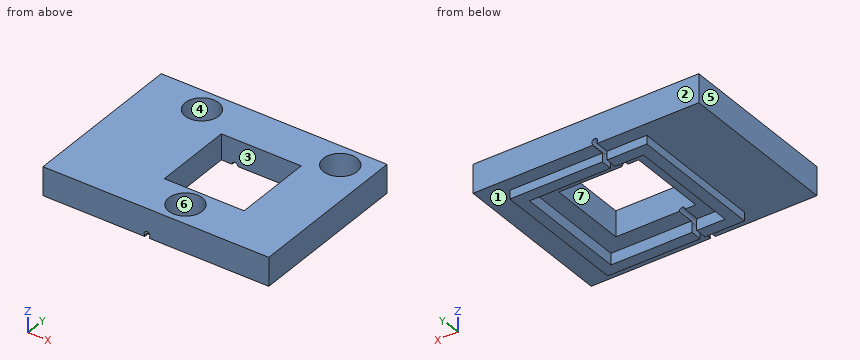
Autodesk Inventor part; units mm, degrees
ref_plane "YZ Plane" through (0, 0, 0) normal (1, 0, 0) x (0, 1, 0)
ref_plane "XZ Plane" through (0, 0, 0) normal (0, 1, 0) x (-1, 0, 0)
ref_plane "XY Plane" through (0, 0, 0) normal (0, 0, 1) x (1, 0, 0)
ref_plane "Work Plane1" through (52.5141, 202.7033, 6.4479) normal (0, 0, -1) x (0, 1, 0)
sketch "Sketch1" plane through (52.5141, 202.7033, 6.4479) normal (0, 0, -1) x (0, 1, 0)
  circle A0 centre (-59.8114, -30.5) radius 1.4 construction
  circle A1 centre (-38.8114, -18.3756) radius 1.4
  circle A2 centre (-38.8114, -42.6244) radius 1.4 construction
  circle A3 centre (41, 0) radius 1.65
  circle A4 centre (-9, 0) radius 1.65
  circle A5 centre (-9, 50) radius 1.65
  circle A6 centre (41, 50) radius 1.65
  circle A7 centre (16, 50) radius 1.65
  circle A8 centre (-9, 25) radius 1.65
  circle A9 centre (16, 0) radius 1.65
  circle A10 centre (41, 25) radius 1.65
  line L0 (80, 55) -> (-80, 55)
  line L1 (-80, 55) -> (-80, -55)
  line L2 (-80, -55) -> (80, -55)
  line L3 (80, -55) -> (80, 55)
  line L4 (-36.5, 0) -> (-36.5, -50)
  line L5 (-14, 0) -> (-36.5, 0)
  line L6 (-14, -5) -> (-14, 0)
  line L7 (72, -5) -> (-14, -5)
  line L8 (72, -50) -> (72, -5)
  line L9 (-36.5, -50) -> (72, -50)
  line L10 (-4, 45) -> (-4, 5)
  line L11 (36, 45) -> (-4, 45)
  line L12 (36, 5) -> (36, 45)
  line L13 (-4, 5) -> (36, 5)
  line L14 (-64.5989, -17.0433) -> (-64.5989, -57.0433) construction
  line L15 (-64.5989, -57.0433) -> (-34.5989, -57.0433) construction
  line L16 (-34.5989, -57.0433) -> (-34.5989, -17.0433) construction
  line L17 (-34.5989, -17.0433) -> (-64.5989, -17.0433) construction
  line L18 (-34.8114, -13.0433) -> (-63.8114, -13.0433)
  line L19 (-63.8114, -13.0433) -> (-63.8114, -52.6244)
  line L20 (-63.8114, -52.6244) -> (-34.8114, -52.6244)
  line L21 (-34.8114, -52.6244) -> (-34.8114, -13.0433)
  circle A11 centre (-59.8114, -30.5) radius 2.95
  circle A12 centre (-38.8114, -18.3756) radius 2.95
  circle A13 centre (-38.8114, -42.6244) radius 2.95 construction
  line L22 (-36.5, -35.1157) -> (-41.75, -35.1157) construction
  line L23 (-41.75, -35.1157) -> (-41.75, -38.5657) construction
  line L24 (-41.75, -38.5657) -> (-56.86, -38.5657) construction
  line L25 (-56.86, -38.5657) -> (-56.86, -35.1157) construction
  line L26 (-56.86, -35.1157) -> (-60.26, -35.1157) construction
  line L27 (-60.26, -35.1157) -> (-60.26, -52.0657) construction
  line L28 (-60.26, -52.0657) -> (-36.5, -52.0657) construction
  line L29 (-36.5, -52.0657) -> (-36.5, -35.1157) construction
  line L30 (-41.75, -28.3657) -> (-36.5, -28.3657) construction
  line L31 (-36.5, -28.3657) -> (-36.5, -25.0657) construction
  line L32 (-36.5, -25.0657) -> (-60.26, -25.0657) construction
  line L33 (-60.26, -25.0657) -> (-60.26, -28.3657) construction
  line L34 (-60.26, -28.3657) -> (-56.86, -28.3657) construction
  line L35 (-56.86, -28.3657) -> (-56.86, -27.0942) construction
  line L36 (-56.86, -27.0942) -> (-41.75, -27.0942) construction
  line L37 (-41.75, -27.0942) -> (-41.75, -28.3657) construction
  line L38 (-56.86, -35.1157) -> (-60.26, -35.1157) construction
  line L39 (-56.86, -38.5657) -> (-56.86, -35.1157) construction
  line L40 (-41.75, -38.5657) -> (-56.86, -38.5657) construction
  line L41 (-41.75, -35.1157) -> (-41.75, -38.5657) construction
  line L42 (-36.5, -35.1157) -> (-41.75, -35.1157) construction
  line L43 (-36.5, -35.05) -> (-36.5, -35.1157) construction
  line L44 (-36.5, -35.05) -> (-56.86, -35.05) construction
  line L45 (-36.5, -34.78) -> (-36.5, -35.05) construction
  line L46 (-36.5, -34.78) -> (-56.86, -34.78) construction
  line L47 (-36.5, -34.51) -> (-36.5, -34.78) construction
  line L48 (-36.5, -34.51) -> (-56.86, -34.51) construction
  line L49 (-36.5, -34.24) -> (-36.5, -34.51) construction
  line L50 (-36.5, -34.24) -> (-56.86, -34.24) construction
  line L51 (-36.5, -33.97) -> (-36.5, -34.24) construction
  line L52 (-36.5, -33.97) -> (-56.86, -33.97) construction
  line L53 (-36.5, -33.7) -> (-36.5, -33.97) construction
  line L54 (-36.5, -33.7) -> (-56.86, -33.7) construction
  line L55 (-36.5, -33.43) -> (-36.5, -33.7) construction
  line L56 (-36.5, -33.43) -> (-56.86, -33.43) construction
  line L57 (-36.5, -33.16) -> (-36.5, -33.43) construction
  line L58 (-36.5, -33.16) -> (-56.86, -33.16) construction
  line L59 (-36.5, -32.89) -> (-36.5, -33.16) construction
  line L60 (-36.5, -32.89) -> (-56.86, -32.89) construction
  line L61 (-36.5, -32.62) -> (-36.5, -32.89) construction
  line L62 (-36.5, -32.62) -> (-56.86, -32.62) construction
  line L63 (-36.5, -32.35) -> (-36.5, -32.62) construction
  line L64 (-36.5, -32.35) -> (-56.86, -32.35) construction
  line L65 (-36.5, -32.08) -> (-36.5, -32.35) construction
  line L66 (-36.5, -32.08) -> (-56.86, -32.08) construction
  line L67 (-36.5, -31.81) -> (-36.5, -32.08) construction
  line L68 (-36.5, -31.81) -> (-56.86, -31.81) construction
  line L69 (-36.5, -31.54) -> (-36.5, -31.81) construction
  line L70 (-36.5, -31.54) -> (-56.86, -31.54) construction
  line L71 (-36.5, -31.27) -> (-36.5, -31.54) construction
  line L72 (-36.5, -31.27) -> (-56.86, -31.27) construction
  line L73 (-36.5, -31) -> (-36.5, -31.27) construction
  line L74 (-36.5, -31) -> (-56.86, -31) construction
  line L75 (-36.5, -30.73) -> (-36.5, -31) construction
  line L76 (-36.5, -30.73) -> (-56.86, -30.73) construction
  line L77 (-36.5, -30.46) -> (-36.5, -30.73) construction
  line L78 (-36.5, -30.46) -> (-56.86, -30.46) construction
  line L79 (-36.5, -30.19) -> (-36.5, -30.46) construction
  line L80 (-36.5, -30.19) -> (-56.86, -30.19) construction
  line L81 (-36.5, -29.92) -> (-36.5, -30.19) construction
  line L82 (-36.5, -29.92) -> (-56.86, -29.92) construction
  line L83 (-36.5, -29.65) -> (-36.5, -29.92) construction
  line L84 (-36.5, -29.65) -> (-56.86, -29.65) construction
  line L85 (-36.5, -29.38) -> (-36.5, -29.65) construction
  line L86 (-36.5, -29.38) -> (-56.86, -29.38) construction
  line L87 (-36.5, -29.11) -> (-36.5, -29.38) construction
  line L88 (-36.5, -29.11) -> (-56.86, -29.11) construction
  line L89 (-36.5, -28.84) -> (-36.5, -29.11) construction
  line L90 (-36.5, -28.84) -> (-56.86, -28.84) construction
  line L91 (-36.5, -28.3657) -> (-36.5, -28.84) construction
  line L92 (-41.75, -28.3657) -> (-36.5, -28.3657) construction
  line L93 (-41.75, -27.0942) -> (-41.75, -28.3657) construction
  line L94 (-56.86, -27.0942) -> (-41.75, -27.0942) construction
  line L95 (-56.86, -28.3657) -> (-56.86, -27.0942) construction
  line L96 (-60.26, -28.3657) -> (-56.86, -28.3657) construction
  line L97 (-60.26, -35.1157) -> (-60.26, -28.3657) construction
  line L98 (-60.26, -25.0657) -> (-36.5, -25.0657) construction
  line L99 (-36.5, -25.0657) -> (-36.5, -52.0657) construction
  line L100 (-60.26, -52.0657) -> (-60.26, -25.0657) construction
  line L101 (-57.1632, -22.5233) -> (-33.4032, -22.5233) construction
  line L102 (-33.4032, -22.5233) -> (-33.4032, -49.5233) construction
  line L103 (-33.4032, -49.5233) -> (-57.1632, -49.5233) construction
  line L104 (-57.1632, -49.5233) -> (-57.1632, -22.5233) construction
  circle A14 centre (-38.8114, -42.6244) radius 2.95
  point P0 (-202.7033, -52.5141)
  point P1 (-56.7146, -27.9576)
  dimension "d0" = 4
  dimension "d2" = 4
  dimension "d3" = 4
  dimension "d4" = 5.9
  dimension "d5" = 5.9
  dimension "d6" = 5.9
  dimension "d10" = 10
extrude "Extrusion1" add sketch "Sketch1" along normal blind 2.5 contours L18 L21 L9 L4 A14 A12 | L4 A12 A14 L9 L21 L20 L19 L18
sketch "Sketch2" plane through (52.5141, 202.7033, 3.9479) normal (0, 0, -1) x (-1, 0, 0)
  circle A0 centre (42.6244, -38.8114) radius 2.95
  circle A1 centre (18.3756, -38.8114) radius 2.95
  circle A2 centre (30.5, -59.8114) radius 2.95
  line L0 (13.0433, -34.8114) -> (13.0433, -63.8114)
  line L1 (13.0433, -63.8114) -> (52.6244, -63.8114)
  line L2 (52.6244, -63.8114) -> (52.6244, -34.8114)
  line L3 (52.6244, -34.8114) -> (13.0433, -34.8114)
  point P0 (52.5141, -202.7033)
extrude "Extrusion2" add sketch "Sketch2" along normal blind 2.5 contours A0 | A1 | A2 | L3 L2 L1 L0
sketch "Sketch6" plane through (52.5141, 202.7033, 1.4479) normal (0, 0, -1) x (-1, 0, 0)
  line L0 (13.0433, -34.8114) -> (13.0433, -63.8114)
  line L1 (13.0433, -63.8114) -> (52.6244, -63.8114)
  line L2 (52.6244, -63.8114) -> (52.6244, -34.8114)
  line L3 (52.6244, -34.8114) -> (13.0433, -34.8114)
  line L4 (36.772, -42.2392) -> (22.772, -42.2392)
  line L5 (22.772, -42.2392) -> (22.772, -56.2392)
  line L6 (22.772, -56.2392) -> (36.772, -56.2392)
  line L7 (36.772, -56.2392) -> (36.772, -42.2392)
  point P0 (52.5141, -202.7033)
  dimension "d33" = 14
  dimension "d34" = 14
extrude "Extrusion6" cut sketch "Sketch6" against normal through all contours L7 L6 L5 L4
sketch "Sketch7" plane through (52.5141, 202.7033, 1.4479) normal (0, 0, -1) x (-1, 0, 0)
  line L0 (22.772, -56.2392) -> (22.772, -42.2392)
  line L1 (22.772, -42.2392) -> (36.772, -42.2392)
  line L2 (36.772, -42.2392) -> (36.772, -56.2392)
  line L3 (36.772, -56.2392) -> (22.772, -56.2392)
  line L4 (13.0433, -34.8114) -> (13.0433, -63.8114)
  line L5 (13.0433, -63.8114) -> (52.6244, -63.8114)
  line L6 (52.6244, -63.8114) -> (52.6244, -34.8114)
  line L7 (52.6244, -34.8114) -> (13.0433, -34.8114)
  line L8 (39.772, -59.2392) -> (39.772, -39.2392)
  line L9 (39.772, -39.2392) -> (19.772, -39.2392)
  line L10 (19.772, -39.2392) -> (19.772, -59.2392)
  line L11 (19.772, -59.2392) -> (39.772, -59.2392)
  point P0 (52.5141, -202.7033)
  dimension "d37" = 20
extrude "Extrusion7" cut sketch "Sketch7" against normal blind 0.5 contours L11 L10 L9 L8
sketch "Sketch8" plane through (52.5141, 202.7033, 1.4479) normal (0, 0, -1) x (-1, 0, 0)
  line L0 (19.772, -39.2392) -> (39.772, -39.2392)
  line L1 (39.772, -39.2392) -> (39.772, -59.2392)
  line L2 (39.772, -59.2392) -> (19.772, -59.2392)
  line L3 (19.772, -59.2392) -> (19.772, -39.2392)
  line L4 (13.0433, -34.8114) -> (13.0433, -63.8114)
  line L5 (13.0433, -63.8114) -> (52.6244, -63.8114)
  line L6 (52.6244, -63.8114) -> (52.6244, -34.8114)
  line L7 (52.6244, -34.8114) -> (13.0433, -34.8114)
  line L8 (41.772, -61.2392) -> (41.772, -37.2392)
  line L9 (41.772, -37.2392) -> (17.772, -37.2392)
  line L10 (17.772, -37.2392) -> (17.772, -61.2392)
  line L11 (17.772, -61.2392) -> (41.772, -61.2392)
  point P0 (52.5141, -202.7033)
  dimension "d40" = 2
extrude "Extrusion8" add sketch "Sketch8" along normal blind 1.5 contours L11 L10 L9 L8
sketch "Sketch9" plane through (-0.1103, 138.8919, 6.4479) normal (0, -1, 0) x (1, 0, 0)
  line L0 (12.8524, -4.5) -> (32.8524, -4.5)
  line L1 (34.8524, -6.5) -> (10.8524, -6.5)
  arc A0 (18.6327, -4.7963) -> (17.8272, -4.7963) centre (18.2299, -4.5) ccw
  line L2 (18.6327, -4.7963) -> (17.8272, -4.7963)
  line L3 (17.8272, -4.7963) -> (17.8272, -6.9787)
  line L4 (17.8272, -6.9787) -> (18.6327, -6.9787)
  line L5 (18.6327, -6.9787) -> (18.6327, -4.7963)
  point P0 (0.1103, -6.4479)
  dimension "d43" = 1
extrude "Extrusion9" cut sketch "Sketch9" against normal through all
sketch "Sketch10" plane through (52.5141, 202.7033, 6.4479) normal (0, 0, 1) x (1, 0, 0)
  circle A0 centre (-42.6244, -38.8114) radius 2.95
  circle A1 centre (-30.5, -59.8114) radius 2.95
  circle A2 centre (-18.3756, -38.8114) radius 2.95
  point P0 (-52.5141, -202.7033)
extrude "Extrusion10" cut sketch "Sketch10" against normal blind 4
properties part number "cellSTORM_v5_chiptray_old_0"
Read the model definition and answer for the solid it produces. Units are mm, in the model's axes. Face numbers are marked on the shaded views. A direction names the side the tool comes from. Give positions to 0.01 mm unless a question says otherwise; leave off trailing zeros. Write each loop counter-clockwise with the first axis right and the second up, starting at its lowest first coordinate (ties: lowest second). Pieces come first, ordered by that corner, then holes. Notation, with made-up numbers: (76.5, -1.5) -> (90.5, -1.5) arc R19 cw to (90.5, 27.5) -> close; hole circle Ø1 at (76, 55.5). An arc over 180 degrees is marked (long way). Answer as a JSON object with one key per item and string values. Group by question number.
1) A tool of negligible diameter and unlimited length cuts with its end or side. For the marked faces 5, 6 and 7, from which of +Z, -Z, +X, -X, +Y, -Y can it reach the whole face along a straight path? Write none if from no direction.
2) Find section A-A (z = 1). Write down the section's boundary in (x, y), and give its area (3 significant figures).
3) Find section D-D (z = 5). Write down the section's boundary in (x, y).
4) Consider L1, parallel to X at y = 156, z = 5.75; L2, parallel to X at y = 164.5, z = 3.25; L3, parallel to Y at x = 17, z = 4.5. Determine where each line is inside the solid, lowest interval first. Write a range as from..to.
5) Find section C-C (y = 141). Write down the section's boundary in (x, z).
6) Find section B-B (x = 27.5). Write down the section's boundary in (y, z).
7) Each of these flat-tipped pins is pushed along its axis until it touches: P1, Ø8, axis at x = 31.5, y = 152, coming from the -Z side; P2, Ø4.5, axis at x = 34.14, y = 163.89, coming from the +Z side; P3, Ø0.8, axis at x = 29, z = 1, coming from the +Y side. Where does it stop, or does it pass through?
8) The mould has two halves that part along Y. Classify the marked faces 1, 2, 3 and 4: +Y half, -Y half, draft (parallel to the pull), parting line (faces both ways), or undercut.
Values follow:
{
 "1": {"face 5": "+Z, -Z, -X, +Y, -Y", "face 6": "+Z", "face 7": "+Z, -Z"},
 "2": {"outline": "(10.74, 141.46) -> (17.72, 141.46) -> (17.72, 143.46) -> (12.74, 143.46) -> (12.74, 163.46) -> (17.72, 163.46) -> (17.72, 165.46) -> (10.74, 165.46) -> close; (18.52, 141.46) -> (34.74, 141.46) -> (34.74, 165.46) -> (18.52, 165.46) -> (18.52, 163.46) -> (32.74, 163.46) -> (32.74, 143.46) -> (18.52, 143.46) -> close", "area": "173 mm2"},
 "3": {"outline": "(-0.11, 138.89) -> (39.47, 138.89) -> (39.47, 167.89) -> (-0.11, 167.89) -> close; hole circle Ø5.9 at (9.89, 163.89); hole (15.74, 146.46) -> (29.74, 146.46) -> (29.74, 160.46) -> (15.74, 160.46) -> close; hole circle Ø5.9 at (22.01, 142.89); hole circle Ø5.9 at (34.14, 163.89)"},
 "4": {"L1": "x = -0.11..15.74, 29.74..39.47", "L2": "x = -0.11..7, 12.78..31.25, 37.03..39.47", "L3": "y = 138.89..146.46, 160.46..167.89"},
 "5": {"outline": "(-0.11, 1.45) -> (17.72, 1.45) -> (17.72, 1.65) arc R0.5 cw (long way) to (18.52, 1.65) -> (18.52, 1.45) -> (39.47, 1.45) -> (39.47, 6.45) -> (24.28, 6.45) -> (24.28, 2.45) -> (19.75, 2.45) -> (19.75, 6.45) -> (-0.11, 6.45) -> close"},
 "6": {"outline": "(138.89, 1.45) -> (141.46, 1.45) -> (141.46, -0.05) -> (143.46, -0.05) -> (143.46, 1.95) -> (146.46, 1.95) -> (146.46, 6.45) -> (138.89, 6.45) -> close; (160.46, 1.95) -> (163.46, 1.95) -> (163.46, -0.05) -> (165.46, -0.05) -> (165.46, 1.45) -> (167.89, 1.45) -> (167.89, 6.45) -> (160.46, 6.45) -> close"},
 "7": {"P1": "stops at z = -0.05", "P2": "stops at z = 2.45", "P3": "stops at y = 165.46"},
 "8": {"face 1": "draft", "face 2": "+Y half", "face 3": "undercut", "face 4": "undercut"}
}
